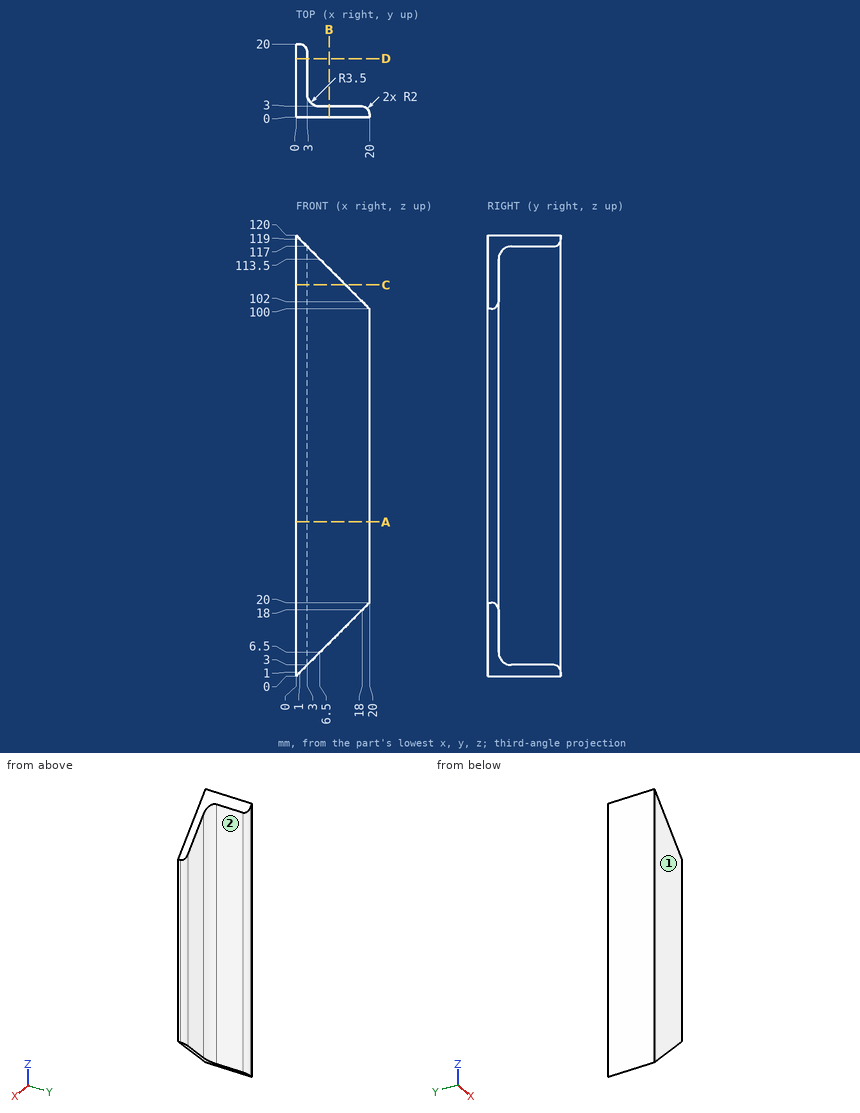
Verification items for this drawing (mm, ordinates from the low corner). A direction names the side the tool comes from. Give positions to 0.01 mm unless a question says otherwise; leave off trailing zeros. Loops run counter-clockwise (first coordinate to the right, second up) from the corner with the lowest first, then second, coordinate; pieces in that order, holes last. Notation, with made-up numbers: M 76.5,76.5 L 124.5,76.5 A24 ccw 124.5,110.5 Z; hole C 60,20 d1. An arc over 180 degrees is marked long. Answer as a JSON object with one key per item and string values. Group by question number.
Item 1: Sectioned sample at C-C on z = 106.5. Record the boundary of the cut face in (x, y), plus the area to 3 significant figures.
Item 2: Material ranges on L1, parallel to Y at x = 14, z = 18; L2, parallel to Z at x = 18, y = 2.25, recorded low to high.
Item 3: Gauge pin test, flat ends, axial feed: pin 1 (2 mm diameter, centred on x = 3.5, y = 2.5, fed in from -Z); pin 2 (2 mm diameter, centred on x = 7, z = 86, fed in from +Y); pin 3 (5 mm diameter, centred on x = 7, y = 7.5, fed in from -Z); pin 4 (3.5 mm diameter, centred on y = 14, z = 87, fed in from +X). Record the tip position at first contact, or that the pin passes through.
Item 4: Sectioned sample at B-B on x = 9. Record the boundary of the cut face in (y, z).
Item 5: Access from +Z, -Z, +X, -X, +Y, -Y to the whole of each face (thin tool, end or side, straight path). Record for the marked faces 1 and 2.
Item 6: Sectioned sample at A-A on z = 42. Record the boundary of the cut face in (x, y).
Item 7: Sectioned sample at D-D on y = 16. Record the boundary of the cut face in (x, z).
Findings below:
{
 "1": {"outline": "M 0,0 L 13.5,0 L 13.5,3 L 6.5,3 A3.5 cw 3,6.5 L 3,18 A2 ccw 1,20 L 0,20 Z", "area": "93.3 mm2"},
 "2": {"L1": "0 to 3", "L2": "18 to 102"},
 "3": {"pin 1": "z = 2.5", "pin 2": "y = 3.04", "pin 3": "through", "pin 4": "x = 3"},
 "4": {"outline": "M 0,9 L 3,9 L 3,111 L 0,111 Z"},
 "5": {"face 1": "+Z, -Z, +X, -X, -Y", "face 2": "+Z, -Z, +X, +Y"},
 "6": {"outline": "M 0,0 L 20,0 L 20,1 A2 ccw 18,3 L 6.5,3 A3.5 cw 3,6.5 L 3,18 A2 ccw 1,20 L 0,20 Z"},
 "7": {"outline": "M 0,0 L 3,3 L 3,117 L 0,120 Z"}
}
